Geometry: final body of the model. Coordinates: model frame, mm. A direction names the side the tool comes from. Give positions to 0.01 mm unless a question says otherwise; leave off trailing zeros. Write each loop counter-clockwise with the first axis right and the second up, starting at its lowest first coordinate (ties: lowest second). Pieces come first, ordered by that corner, then holes. Notation, with made-up numbers: (-13.5, 20.5) -> (13.5, 20.5) arc R36 cw to (13.5, 57.5) -> close; hole circle Ø2 at (-33, -25). An arc over 180 degrees is marked (long way). Answer in a Markdown table with one row per item. Add a question column.
Item 1: Access query for faces 1 (the flat face through (0, 0, -10)), 2 (the flat face through (-0.49, 0.87, 1.16)). Directions: +Z, -Z, +X, -X, +Y, -Y. A direction counts if a zero-diameter tool reaches every point of the face in a straight line with its end or side. Return the directions, or none.
Item 2: Section query A-A on z = -1.5. Output: boundary loops of the cut face in (x, y).
Item 3: Material intervals for probe 1 along Z at (x, y) = (-0.2, -0.7); probe 2 along X at (y, z) = (-0.1, -3); probe 3 along Y at (x, z) = (-0.75, 0.25), sorted ascending. Write a range as from..to.
Item 4: Draft query along X for faces 3 (the flat face through (1, 0, 1)), 4 (the cylindrical face through (0.07, -1.5, -4.97)), 5 (the flat face through (-1.2, 1.2, 0)), 6 (the flat face through (0.51, 0.86, 1.16)). Return one class per face: +X half, -X half, draft (parallel to the pull), parting line (faces both ways), or undercut.
Item 5: First-contact query: P1, Ø0.5, axis at y = 0, z = 1.5, coming from the -X side; P2, Ø2, axis at x = 1.5, z = -3.5, coming from the +Y side; P3, Ø2, axis at x = -0.5, z = -6.5, coming from the +Y side. Flat tips, straight axial feed; report the tip coordinate or a pass-through.
```python
from build123d import *

# Parameters (mm, degrees)
CORTAR_EXTRUIR2_DEPTH = 1
CHAFL_N1_SIZE         = 0.2


with BuildPart() as part:
    # Croquis1 → Revolución1 (revolve)
    with BuildSketch(Plane(origin=(0, 0, 0), x_dir=(0, 0, -1), z_dir=(1, 0, 0))):
        with BuildLine():
            Line((0, 2.85), (0, 1.5))
            Line((0, 1.5), (10, 1.5))
            Line((10, 1.5), (10, 0))
            Line((10, 0), (-1.65, 0))
            Line((-1.65, 0), (-1.65, 1.5))
            ThreePointArc((-1.65, 1.5), (-0.955984269, 2.335091885), (0, 2.85))
        make_face()
    revolve(axis=Axis((0, 0, -10), (0, 0, -1)))

    # Croquis2 → Cortar-Extruir2 (cut)
    with BuildSketch(Plane.XY.offset(1.65)):
        Polygon((0, 1.154700538), (-1, 0.577350269), (-1, -0.577350269), (0, -1.154700538), (1, -0.577350269), (1, 0.577350269), align=None)
    extrude(amount=-CORTAR_EXTRUIR2_DEPTH, mode=Mode.SUBTRACT)

    # Chaflán1
    chafl_n1_edges = [part.edges().sort_by_distance(p)[0] for p in [
        (0, -1.5, -10),
    ]]
    chamfer(chafl_n1_edges, length=CHAFL_N1_SIZE)


solid = part.part
```
Findings below:
| question | item | result |
|---|---|---|
| 1 | face 1 | -Z, +X, -X, +Y, -Y |
| 1 | face 2 | +Z |
| 2 | outline | circle Ø3 at (0, 0) |
| 3 | probe 1 | z = -10..0.65 |
| 3 | probe 2 | x = -1.5..1.5 |
| 3 | probe 3 | y = -2.66..2.66 |
| 4 | face 3 | undercut |
| 4 | face 4 | parting line |
| 4 | face 5 | draft |
| 4 | face 6 | undercut |
| 5 | P1 | stops at x = -2.06 |
| 5 | P2 | stops at y = 1.41 |
| 5 | P3 | stops at y = 1.5 |
